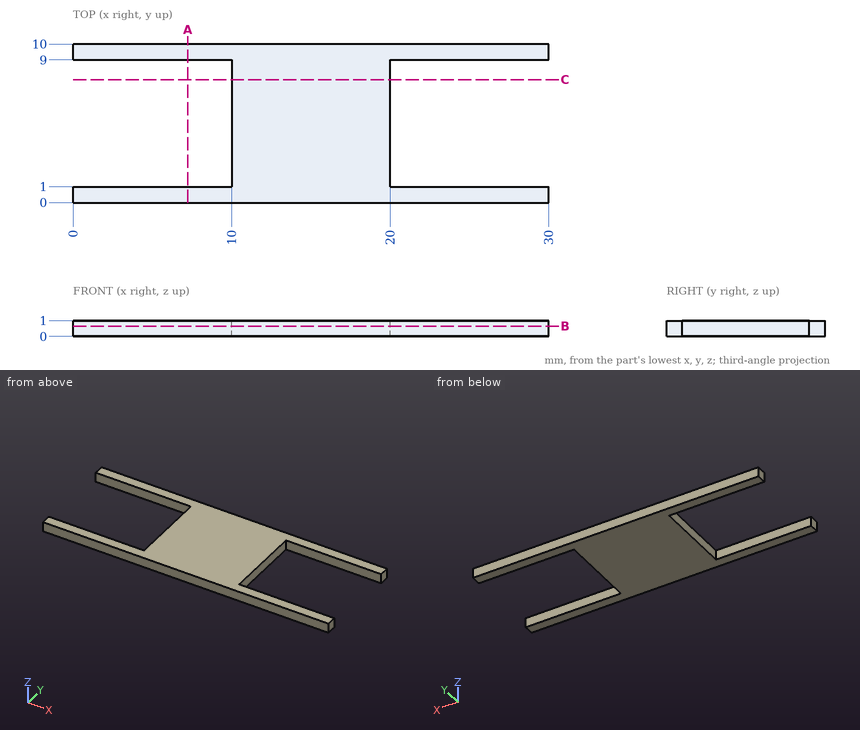
For this review, use the dimensioned drawing (mm, ordinates from the lowest corner) and the shaded views. Coordinates: 2 decimals unless noted, no trailing zeros. Write each loop counter-clockwise with the first axis right and the second up, starting at its lowest first coordinate (ties: lowest second). Pieces come first, ordered by that corner, then holes. Notation, with made-up numbers: (31.5, -19) - (70.5, -19) arc R6 cw to (70.5, -11) - close; hole circle Ø3 at (21, 4). An arc over 180 degrees is marked (long way). Answer in a Markdown table with one row per item. Add a question column.
Q1. To check wall thickness, follow line 1 along Y through (x, z) = (26.5, 0.3); line 2 along X through (y, z) = (5.25, 0.35). State the ranges of each line that lie inside material, in increasing order. Write a range as from..to.
Q2. Consider section C-C on y = 7.75. Give the boundary of the cut face in (x, z), then the cut area to 3 significant figures.
Q3. Consider section B-B on z = 0.65. Give the boundary of the cut face in (x, y).
Q4. Consider section A-A on x = 7.25. Give the boundary of the cut face in (y, z), then the cut area to 3 significant figures.
Q5. Clearance check with a flat-ended pin moving along its axis: pin 1 (0.5 mm diameter, centred on y = 4.5, z = 0.5, fed in from -X). State where the tip first meets the part, or that it passes through.
Answers below:
| question | item | result |
|---|---|---|
| 1 | line 1 | 0..1, 9..10 |
| 1 | line 2 | 10..20 |
| 2 | outline | (10, 0) - (20, 0) - (20, 1) - (10, 1) - close |
| 2 | area | 10.0 mm² |
| 3 | outline | (0, 0) - (30, 0) - (30, 1) - (20, 1) - (20, 9) - (30, 9) - (30, 10) - (0, 10) - (0, 9) - (10, 9) - (10, 1) - (0, 1) - close |
| 4 | outline | (0, 0) - (1, 0) - (1, 1) - (0, 1) - close; (9, 0) - (10, 0) - (10, 1) - (9, 1) - close |
| 4 | area | 2.00 mm² |
| 5 | pin 1 | x = 10 |
